Part model, mm, in its own coordinate system. A direction names the side the tool comes from. Coordinates: 2 decimals unless noted, no trailing zeros. Write each loop counter-clockwise with the first axis right and the second up, starting at its lowest first coordinate (ties: lowest second). Pieces come first, ordered by that corner, then holes. Notation, with made-up numbers: M 21,38 L 67,38 A21 cw 67,65 Z; hole C 70.25,-9.75 d8. An arc over 180 degrees is marked long. Use a Markdown table: item, result. Add a question column.
Q1. Wall check: L1, parallel to Z at x = 117, y = 8.89; L2, parallel to Y at x = 112.75, z = -6.35; L3, parallel to X at y = 22, z = -3.5. Give the ranges that are in metal, low to high. Write a range as from..to.
Q2. Tool access for faces 4 (the flat face through (4.25, 18.96, -6.26)), 5 (the flat face through (81, 17.78, -6)), 6 (the flat face through (60, 10, 0)): list every direction of +Z, -Z, +X, -X, +Y, -Y with a clear straight run to the whole face (end or side of a thin tool).
Q3. Slice it at C-C on y = 23.25. Write the cut outline in (x, z).
Q4. Slice it at B-B on x = 78.5. Write the cut outline in (y, z).
Q5. Pin check, flat tips, straight feed: pin 1 Ø1.5 at (y, z) = (20, -5) entering from +X; pin 2 Ø0.7 at (x, z) = (1.5, -4.5) entering from +Y; pin 3 Ø4 at (y, z) = (8.89, -6.35) entering from +X; pin 4 Ø4 at (y, z) = (9, -7) entering from +X. Stop position of each tip, or through.
Q6. Slice it at A-A on y = 8.89. Write the cut outline in (x, z), then the cut area to 3 significant figures.
Q7. Mould opens along Y. For faces 1 (the flat face through (107.95, 9, -6)), 2 (the flat face through (60, 10, -12.7)), 3 (the flat face through (35.659, 18.928, -6.261)) say: released by +Y, released by -Y, zero draft, split by the parting line, or undercut.
from build123d import *

# Parameters (mm, degrees)
BLANKSKE_W          = 76.2
BLANKSKE_H          = 20.108333333
BLANK_DEPTH         = 12.7
TOOTHCUTSIM_DEPTH   = 80.825278386
TEETHCUTS_COUNT     = 24
TEETHCUTS_PITCH     = 3.324852221
SKETCH1_W           = 12.7
SKETCH1_H           = 17.78
BOSS_EXTRUDE1_DEPTH = 44.45
SKETCH3_R           = 2.54
CUT_EXTRUDE1_DEPTH  = 12.7
SKETCH4_W           = 0.496986858
SKETCH4_H           = 12.7
BOSS_EXTRUDE2_DEPTH = 7.62
SKETCH5_W           = 12.7
SKETCH5_H           = 25.4
BOSS_EXTRUDE3_DEPTH = 2.032
SKETCH6_W           = 12.7
SKETCH6_H           = 2.328333333
CUT_EXTRUDE2_DEPTH  = 76.962


with BuildPart() as part:
    # BlankSke → Blank (new body)
    with BuildSketch(Plane.XY):
        with Locations((38.1, 10.054166667)):
            Rectangle(BLANKSKE_W, BLANKSKE_H)
    extrude(amount=-BLANK_DEPTH)

    # TooCutSkeSim → ToothCutSim (cut, through all)
    with BuildSketch(Plane.XY):
        Polygon((0.496986858, 17.78), (-0.496986858, 17.78), (-1.353675731, 20.133733333), (1.353675731, 20.133733333), align=None)
    toothcutsim = extrude(amount=-TOOTHCUTSIM_DEPTH, mode=Mode.SUBTRACT)

    # TeethCuts: ToothCutSim ×24
    with Locations(*[(i * TEETHCUTS_PITCH, 0, 0) for i in range(1, TEETHCUTS_COUNT)]):
        add(toothcutsim, mode=Mode.SUBTRACT)

    # Sketch1 → Boss-Extrude1 (add)
    with BuildSketch(Plane(origin=(76.2, 0, 0), x_dir=(0, 0, -1), z_dir=(1, 0, 0))):
        with Locations((6.35, 8.89)):
            Rectangle(SKETCH1_W, SKETCH1_H)
    extrude(amount=BOSS_EXTRUDE1_DEPTH)

    # Sketch3 → Cut-Extrude1 (cut)
    with BuildSketch(Plane(origin=(120.65, 0, -120.65), x_dir=(0, 0, 1), z_dir=(-1, 0, 0))):
        with Locations(Location((114.3, 8.89, 0), (0, 0, 90))):
            Circle(SKETCH3_R)
    extrude(amount=CUT_EXTRUDE1_DEPTH, mode=Mode.SUBTRACT)

    # Sketch4 → Boss-Extrude2 (add)
    with BuildSketch(Plane(origin=(0, 17.78, 0), x_dir=(1, 0, 0), z_dir=(0, 1, 0))):
        with Locations((0.248493429, 6.35)):
            Rectangle(SKETCH4_W, SKETCH4_H)
    extrude(amount=BOSS_EXTRUDE2_DEPTH)

    # Sketch5 → Boss-Extrude3 (add)
    with BuildSketch(Plane.ZY):
        with Locations((-6.35, 12.7)):
            Rectangle(SKETCH5_W, SKETCH5_H)
    extrude(amount=BOSS_EXTRUDE3_DEPTH)

    # Sketch6 → Cut-Extrude2 (cut)
    with BuildSketch(Plane(origin=(120.65, 0, 0), x_dir=(0, 0, -1), z_dir=(1, 0, 0))):
        with Locations((6.35, 18.944166667)):
            Rectangle(SKETCH6_W, SKETCH6_H)
    extrude(amount=-CUT_EXTRUDE2_DEPTH, mode=Mode.SUBTRACT)


solid = part.part
Recorded:
| question | item | result |
|---|---|---|
| 1 | L1 | -12.7..-8.89, -3.81..0 |
| 1 | L2 | 0..6.35, 11.43..17.78 |
| 1 | L3 | -2.03..0.5 |
| 2 | face 4 | +Z, -Z, +Y |
| 2 | face 5 | +Z, -Z, +X, +Y |
| 2 | face 6 | +Z, +X, -X, +Y, -Y |
| 3 | outline | M -2.03,-12.7 L 0.5,-12.7 L 0.5,0 L -2.03,0 Z |
| 4 | outline | M 0,-12.7 L 17.78,-12.7 L 17.78,0 L 0,0 Z |
| 5 | pin 1 | x = 42.19 |
| 5 | pin 2 | y = 20.11 |
| 5 | pin 3 | x = 107.95 |
| 5 | pin 4 | x = 120.65 |
| 6 | outline | M -2.03,-12.7 L 120.65,-12.7 L 120.65,-8.89 L 107.95,-8.89 L 107.95,-3.81 L 120.65,-3.81 L 120.65,0 L -2.03,0 Z |
| 6 | area | 1,490 mm² |
| 7 | face 1 | undercut |
| 7 | face 2 | zero draft |
| 7 | face 3 | released by +Y |
